from build123d import *

# Parameters (mm, degrees)
BOSS_EXTRUDE1_DEPTH = 58
SKETCH5_R           = 7
CUT_EXTRUDE1_DEPTH  = 116.341103519
SKETCH7_R           = 7
CUT_EXTRUDE2_DEPTH  = 116.341103519
CUT_EXTRUDE3_DEPTH  = 116.341103519
CUT_EXTRUDE4_DEPTH  = 116.341103519


with BuildPart() as part:
    # Sketch1 → Boss-Extrude1 (new body)
    with BuildSketch(Plane.XY):
        Polygon((0, 0), (65, 0), (79.621417728, 14.621417728), (79.621417728, 45.378582272), (65, 60), (0, 60), (0, 52), (13.686014712, 52), (13.686014712, 46), (54, 46), (54, 14), (13.686014712, 14), (13.686014712, 8), (0, 8), align=None)
    extrude(amount=BOSS_EXTRUDE1_DEPTH)

    # Sketch5 → Cut-Extrude1 (cut, through all)
    with BuildSketch(Plane(origin=(79.621417728, 0, 0), x_dir=(0, 0, -1), z_dir=(1, 0, 0))):
        with Locations((-29, 30)):
            Circle(SKETCH5_R)
    extrude(amount=-CUT_EXTRUDE1_DEPTH, mode=Mode.SUBTRACT)

    # Sketch7 → Cut-Extrude2 (cut, through all)
    with BuildSketch(Plane(origin=(0, 60, 0), x_dir=(1, 0, 0), z_dir=(0, 1, 0))):
        with Locations(Location((32.5, -29, 0), (0, 0, 180))):
            Circle(SKETCH7_R)
    extrude(amount=-CUT_EXTRUDE2_DEPTH, mode=Mode.SUBTRACT)

    # Sketch9 → Cut-Extrude3 (cut, through all)
    with BuildSketch(Plane(origin=(0, 0, 0), x_dir=(1, 0, 0), z_dir=(0, 1, 0))):
        Polygon((65, 0), (79.621417728, 0), (79.621417728, -14.621417728), align=None)
        Polygon((65, -58), (79.621417728, -43.378582272), (79.621417728, -58), align=None)
    extrude(amount=CUT_EXTRUDE3_DEPTH, mode=Mode.SUBTRACT)

    # Sketch11 → Cut-Extrude4 (cut, through all)
    with BuildSketch(Plane(origin=(0, 60, 0), x_dir=(1, 0, 0), z_dir=(0, 1, 0))):
        with BuildLine():
            Line((36.71635628, 0), (0, 0))
            Line((0, 0), (0, -17.954880359))
            ThreePointArc((0, -17.954880359), (16.439804094, -5.054512065), (36.71635628, 0))
        make_face()
    extrude(amount=-CUT_EXTRUDE4_DEPTH, mode=Mode.SUBTRACT)


solid = part.part
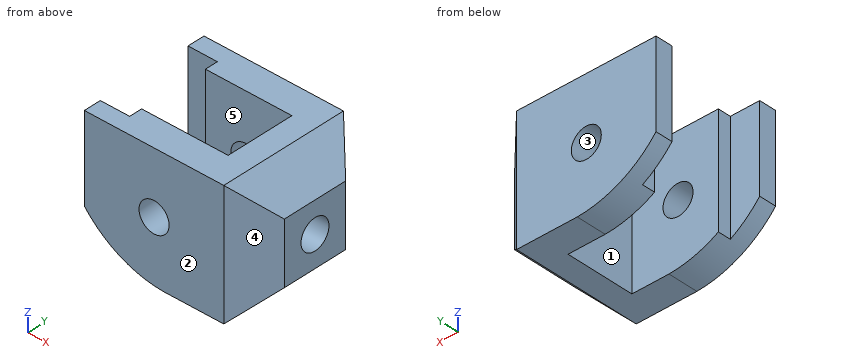
CAD build for the part. Positions are in the model's coordinates, mm. Face numbers are marked on the shaded views. A direction names the side the tool comes from. Round coordinates to 2 decimals unless told otherwise and drop trailing zeros. Loops run counter-clockwise (first coordinate to the right, second up) from the corner with the lowest first, then second, coordinate; pieces in that order, holes last.
(1) Cut at C-C (y = 9.5). Give the cut face in (x, z).
(2) Two-plate mould, pull along X, no slides. Class the marked faces 1, 2 and 3: +X half, -X half, draft (parallel to the pull), parting line (faces both ways), or undercut.
(3) Cut at B-B (z = 54). Give the cut face in (x, y), plus the area to 3 significant figures.
(4) Which spindle directions (+Z, -Z, +X, -X, +Y, -Y) get a long thin tool onto all of the face, cutting with end or side? Do the marked faces 4 and 5. Say none if no direction does.
(5) Wall check: line 1 along Y through (x, z) = (50.5, 10.5); line 2 along Y through (x, z) = (64, 29); line 3 along Z through (x, y) = (37.5, 51.5). Give the ranges that are in metal, low to high.
(6) Cut at D-D (x = 32.5). Give the cut face in (y, z).
(7) Drop flat-ended pins along their axis: pin 1 (2 mm diameter, centred on y = 29.5, z = 50.5, fed in from -X); pin 2 (8 mm diameter, centred on y = 54, z = 6.5, fed in from -X); pin 3 (3 mm diameter, centred on y = 47.5, z = 23, fed in from -X); pin 4 (1.5 mm diameter, centred on x = 32.5, y = 15, fed in from +Z). Give the stop position or say it passes through.
(8) Cut at A-A (y = 30). Give the cut face in (x, z).
Findings below:
1. outline: (13.69, 6.51) arc R50 ccw to (36.72, 0) - (65, 0) - (74.5, 9.5) - (74.5, 48.5) - (65, 58) - (13.69, 58) - close; hole circle Ø14 at (32.5, 29)
2. face 1: -X half
2. face 2: draft
2. face 3: undercut
3. outline: (0, 0) - (65, 0) - (69, 4) - (69, 56) - (65, 60) - (0, 60) - (0, 52) - (13.69, 52) - (13.69, 46) - (54, 46) - (54, 14) - (13.69, 14) - (13.69, 8) - (0, 8) - close
3. area: 2,230 mm2
4. face 4: +Z, -Z, +X, -Y
4. face 5: +Z, -Z, -X
5. line 1: y = 0 to 14, 46 to 60
5. line 2: y = 0 to 23, 37 to 60
5. line 3: z = 0 to 24.1, 33.9 to 58
6. outline: (0, 0.32) - (14, 0.32) - (14, 22) - (0, 22) - close; (0, 36) - (14, 36) - (14, 58) - (0, 58) - close; (46, 0.32) - (60, 0.32) - (60, 22) - (46, 22) - close; (46, 36) - (60, 36) - (60, 58) - (46, 58) - close
7. pin 1: stops at x = 54
7. pin 2: stops at x = 7.71
7. pin 3: stops at x = 13.69
7. pin 4: passes through
8. outline: (54, 0) - (65, 0) - (79.62, 14.62) - (79.62, 22) - (54, 22) - close; (54, 36) - (79.62, 36) - (79.62, 43.38) - (65, 58) - (54, 58) - close
